Autodesk Inventor part; units mm, degrees
ref_plane "YZ Plane" through (0, 0, 0) normal (1, 0, 0) x (0, 1, 0)
ref_plane "XZ Plane" through (0, 0, 0) normal (0, 1, 0) x (-1, 0, 0)
ref_plane "XY Plane" through (0, 0, 0) normal (0, 0, 1) x (1, 0, 0)
sketch "Sketch1" plane through (0, 0, 0) normal (0, 0, 1) x (1, 0, 0)
  line L0 (0, 0) -> (1.8311, 0)
  line L1 (0, 0) -> (0, 45.085)
  line L2 (0.381, 45.085) -> (0.381, 0.381)
  line L3 (0.381, 0.381) -> (1.8311, 0.381)
  line L4 (1.8311, 0.381) -> (1.8311, 0)
  line L5 (0.381, 45.085) -> (0, 45.085)
  dimension "d0" = 1.8311
  dimension "d1" = 45.085
  dimension "d2" = 0.381
extrude "Extrusion1" add sketch "Sketch1" along normal blind 88.9
fillet "Fillet1" radius 2.54 2 edges at (0.1905, 45.085, 88.9) (0.1905, 45.085, 0)
sketch "Sketch2" plane through (0, 0, 0) normal (-1, 0, 0) x (0, 0, 1)
  line L0 (0, 0) -> (88.9, 0)
  circle A0 centre (40.005, 0) radius 3.175
  circle A1 centre (48.895, 0) radius 3.2307
  dimension "d6" = 6.35
  dimension "d7" = 8.89
  dimension "d8" = 40.005
extrude "Extrusion2" cut sketch "Sketch2" against normal blind 88.9
sketch "Sketch3" plane through (0, 0, 0) normal (-1, 0, 0) x (0, 0, 1)
  circle A0 centre (20.32, 31.115) radius 3.4925
  circle A1 centre (68.58, 31.115) radius 3.4925
  line L0 (88.9, 42.545) -> (88.9, 0)
  line L1 (0, 42.545) -> (0, 0)
  line L2 (2.54, 45.085) -> (86.36, 45.085)
  dimension "d11" = 6.985
  dimension "d12" = 6.985
  dimension "d13" = 20.32
  dimension "d14" = 20.32
  dimension "d15" = 13.97
  dimension "d16" = 13.97
extrude "Extrusion3" cut sketch "Sketch3" against normal blind 88.9
sketch "Sketch4" plane through (0, 0, 0) normal (-1, 0, 0) x (0, 0, 1)
  line L0 (88.9, 42.545) -> (88.9, 0)
  line L1 (0, 42.545) -> (0, 0)
  line L2 (2.54, 45.085) -> (86.36, 45.085)
  line L3 (53.6575, 0) -> (72.39, 28.575)
  line L4 (35.2425, 0) -> (16.51, 28.575)
  arc A0 (69.85, 34.925) -> (19.05, 34.925) centre (44.45, -37.6219) ccw
  arc A1 (19.05, 34.925) -> (16.51, 28.575) centre (20.5495, 30.6422) ccw
  arc A2 (72.39, 28.575) -> (69.85, 34.925) centre (68.3505, 30.6422) ccw
  line L5 (35.2425, 0) -> (53.6575, 0)
  line L6 (52.1257, 0) -> (88.9, 0)
  point P0 (44.45, 39.243)
  dimension "d19" = 35.2425
  dimension "d20" = 35.2425
  dimension "d21" = 16.51
  dimension "d22" = 16.51
  dimension "d23" = 16.51
  dimension "d24" = 16.51
  dimension "d25" = 19.05
  dimension "d26" = 19.05
  dimension "d27" = 10.16
  dimension "d28" = 10.16
  dimension "d29" = 5.842
extrude "Extrusion4" cut sketch "Sketch4" against normal blind 25.4
properties part number "Fin_holed" material "Aluminum 6061"
Could you check a few things on this model? Use its own coordinates, in mm. A direction names the side the tool comes from. Round coordinates to 2 decimals unless told otherwise and drop trailing zeros. Loops run counter-clockwise (first coordinate to the right, second up) from the corner with the lowest first, then second, coordinate; pieces in that order, holes last.
Q1. Thinking about a two-plate mould opening in Y: for faces 4 (the flat face through (1, 0, 71)), 5 (the cylindrical face through (0.188, 39.242, 44.812)), 6 (the flat face through (0.2, 21.4, 0)), which applies, pulls with the +Y half, pulls with the -Y half, needs draft (parallel to the pull), parting line crosses it, or undercut?
Q2. On a 3-axis mill with a long thin cutter (end or side, diameter ignored), from which of +Z, -Z, +X, -X, +Y, -Y can I reach the whole of each face in a straight line? I mean faces 1 (the flat face through (1, 0, 17)), 2 (the cylindrical face through (0.188, 32.277, 72.584)), 3 (the flat face through (0.381, 43, 44)). Say none if no direction works.
Q3. I want a section at D-D (z = 79). Write out the boundary of the cut face in (x, y) (3 decimals).
Q4. I want a section at B-B (y = 4). Write out the boundary of the cut face in (x, z), and give its area (3 significant figures).
Q5. I want a section at A-A (x = 0.85). Write out the boundary of the cut face in (y, z).
Q6. Please list where these lines run through material, in increasing order: L1, parallel to Y at x = 0.6, z = 28.5; L2, parallel to Z at x = 0.2, y = 14.
Q7. For P1, Ø6, axis at y = 10.5, z = 33, coming from the -X side; P2, Ø8, axis at y = 14.5, z = 28.5, coming from the +X side; P3, Ø0.7, axis at x = 1, z = 10.5, coming from the +Y side, each with a flat end and sliding along its axis, tell me the tip position at first contact or that it passes through.
Q8. I want a section at C-C (z = 65.5). Write out the boundary of the cut face in (x, y) (3 decimals).
Answer below:
1. face 4: pulls with the -Y half
1. face 5: undercut
1. face 6: needs draft
2. face 1: +Z, -Z, +X, -X, -Y
2. face 2: +X, -X
2. face 3: +Z, -Z, +X, +Y
3. outline: (0, 0) - (1.831, 0) - (1.831, 0.381) - (0.381, 0.381) - (0.381, 45.085) - (0, 45.085) - close
4. outline: (0, 0) - (0.38, 0) - (0.38, 32.62) - (0, 32.62) - close; (0, 56.28) - (0.38, 56.28) - (0.38, 88.9) - (0, 88.9) - close
4. area: 24.9 mm2
5. outline: (0, 0) - (0.38, 0) - (0.38, 34.99) - (0, 35.24) - close; (0, 53.66) - (0.38, 53.91) - (0.38, 88.9) - (0, 88.9) - close
6. L1: y = 0 to 0.38
6. L2: z = 0 to 26.06, 62.84 to 88.9
7. P1: passes through
7. P2: stops at x = 0.38
7. P3: stops at y = 0.38
8. outline: (0, 0) - (1.831, 0) - (1.831, 0.381) - (0.381, 0.381) - (0.381, 18.065) - (0, 18.065) - close; (0, 36.304) - (0.381, 36.304) - (0.381, 45.085) - (0, 45.085) - close
